```python
from build123d import *

# Parameters (mm, degrees)
F0_R     = 1.5
F1_DEPTH = 62
F2_W     = 60.3578643763
F2_H     = 56
F2_W_2   = 59.6421356237
F3_DEPTH = 100
F5_DEPTH = 3
F8_DEPTH = 3


with BuildPart() as f1:
    # F0 (on Front) → F1 (new body)
    with BuildSketch(Plane.XZ):
        with BuildLine():
            ThreePointArc((-3.5355339059, 3.5355339059), (0, 2.0710678119), (3.5355339059, 3.5355339059))
            Line((3.5355339059, 3.5355339059), (44, 44))
            Line((44, 44), (94.5, 44))
            ThreePointArc((94.5, 44), (98.0355339059, 45.4644660941), (99.5, 49))
            Line((99.5, 49), (99.5, 54))
            Line((99.5, 54), (39.8578643763, 54))
            Line((39.8578643763, 54), (-3.5355339059, 10.6066017178))
            ThreePointArc((-3.5355339059, 10.6066017178), (-5, 7.0710678119), (-3.5355339059, 3.5355339059))
        make_face()
        with Locations((0, 7.0710678119)):
            Circle(F0_R, mode=Mode.SUBTRACT)
        with Locations((12, 19.0710678119)):
            Circle(F0_R, mode=Mode.SUBTRACT)
    extrude(amount=F1_DEPTH)

    # F2 (on face) → F3 (cut)
    with BuildSketch(Plane.XY.offset(54)):
        with Locations((9.6789321881, -31)):
            Rectangle(F2_W, F2_H)
        with Locations((69.6789321881, -31)):
            Rectangle(F2_W_2, F2_H)
    extrude(amount=-F3_DEPTH, mode=Mode.SUBTRACT)


with BuildPart() as f5:
    # F4 (on face) → F5 (new body)
    with BuildSketch(Plane.XY.offset(54)):
        with BuildLine():
            ThreePointArc((99.5, -69), (92, -61.5), (84.5, -69))
            ThreePointArc((84.5, -69), (86.0313318068, -73.5414755311), (90, -76.2284161474))
            Line((90, -76.2284161474), (90, -74.123475383))
            ThreePointArc((90, -74.123475383), (88.8975815885, -64.4585244689), (97.5, -69))
            ThreePointArc((97.5, -69), (96.5414755311, -72.1024184115), (94, -74.123475383))
            Line((94, -74.123475383), (94, -76.2284161474))
            ThreePointArc((94, -76.2284161474), (97.9686681932, -73.5414755311), (99.5, -69))
        make_face()
        with BuildLine():
            ThreePointArc((89.3074175964, 0), (85.8175907598, 2.7540824329), (84.5, 7))
            Line((84.5, 7), (84.5, 0))
            Line((84.5, 0), (89.3074175964, 0))
        make_face()
        with BuildLine():
            Line((99.5, -3), (84.5, -3))
            Line((84.5, -3), (84.5, -69))
            ThreePointArc((84.5, -69), (92, -61.5), (99.5, -69))
            Line((99.5, -69), (99.5, -3))
        make_face()
        with BuildLine():
            ThreePointArc((99.5, 7), (98.1824092402, 2.7540824329), (94.6925824036, 0))
            Line((94.6925824036, 0), (99.5, 0))
            Line((99.5, 0), (99.5, 7))
        make_face()
        with BuildLine():
            Line((94.6925824036, 0), (89.3074175964, 0))
            ThreePointArc((89.3074175964, 0), (92, -0.5), (94.6925824036, 0))
        make_face()
        with BuildLine():
            ThreePointArc((90, 14.2284161474), (86.0313318068, 11.5414755311), (84.5, 7))
            ThreePointArc((84.5, 7), (85.8175907598, 2.7540824329), (89.3074175964, 0))
            Line((89.3074175964, 0), (94.6925824036, 0))
            ThreePointArc((94.6925824036, 0), (98.1824092402, 2.7540824329), (99.5, 7))
            ThreePointArc((99.5, 7), (97.9686681932, 11.5414755311), (94, 14.2284161474))
            Line((94, 14.2284161474), (94, 12.123475383))
            ThreePointArc((94, 12.123475383), (96.5414755311, 10.1024184115), (97.5, 7))
            ThreePointArc((97.5, 7), (88.8975815885, 2.4585244689), (90, 12.123475383))
            Line((90, 12.123475383), (90, 14.2284161474))
        make_face()
        with BuildLine():
            Line((89.3074175964, 0), (84.5, 0))
            Line((84.5, 0), (84.5, -3))
            Line((84.5, -3), (99.5, -3))
            Line((99.5, -3), (99.5, 0))
            Line((99.5, 0), (94.6925824036, 0))
            ThreePointArc((94.6925824036, 0), (92, -0.5), (89.3074175964, 0))
        make_face()
    extrude(amount=-F5_DEPTH)


with BuildPart() as f1_1:
    add(f1.part)

    # F6: union F5
    add(f5.part)

    # F7 (on face) → F8 (join)
    with BuildSketch(Plane.XY.offset(54)):
        with BuildLine():
            ThreePointArc((90, 12.123475383), (92, 1.5), (94, 12.123475383))
            Line((94, 12.123475383), (94, 9.8722813233))
            ThreePointArc((94, 9.8722813233), (95.1024184115, 8.6201851746), (95.5, 7))
            ThreePointArc((95.5, 7), (90.3798148254, 3.8975815885), (90, 9.8722813233))
            Line((90, 9.8722813233), (90, 12.123475383))
        make_face()
        with BuildLine():
            ThreePointArc((84.5, 7), (92, -0.5), (99.5, 7))
            ThreePointArc((99.5, 7), (97.9686681932, 11.5414755311), (94, 14.2284161474))
            Line((94, 14.2284161474), (94, 12.123475383))
            ThreePointArc((94, 12.123475383), (92, 1.5), (90, 12.123475383))
            Line((90, 12.123475383), (90, 14.2284161474))
            ThreePointArc((90, 14.2284161474), (86.0313318068, 11.5414755311), (84.5, 7))
        make_face()
        with BuildLine():
            Line((94, -71.8722813233), (94, -74.123475383))
            ThreePointArc((94, -74.123475383), (92, -63.5), (90, -74.123475383))
            Line((90, -74.123475383), (90, -71.8722813233))
            ThreePointArc((90, -71.8722813233), (90.3798148254, -65.8975815885), (95.5, -69))
            ThreePointArc((95.5, -69), (95.1024184115, -70.6201851746), (94, -71.8722813233))
        make_face()
        with BuildLine():
            ThreePointArc((94, -76.2284161474), (97.9686681932, -73.5414755311), (99.5, -69))
            ThreePointArc((99.5, -69), (92, -61.5), (84.5, -69))
            ThreePointArc((84.5, -69), (86.0313318068, -73.5414755311), (90, -76.2284161474))
            Line((90, -76.2284161474), (90, -74.123475383))
            ThreePointArc((90, -74.123475383), (92, -63.5), (94, -74.123475383))
            Line((94, -74.123475383), (94, -76.2284161474))
        make_face()
    extrude(amount=F8_DEPTH)


solid = f1_1.part
```
Verification items for the finished model (mm, model axes). A direction names the side the tool comes from. Round coordinates to 2 decimals unless told otherwise and drop trailing zeros. Order: outer loops, then holes, each group sorted by start corner. A loop starts at its lowest first (then second) coordinate and runs counter-clockwise, first axis right, second up. Notation, with made-up numbers: (60, 14.25) - (115, 14.25) arc R22 cw to (115, 53.25) - close; hole circle Ø1 at (19, 10). An arc over 180 degrees is marked (long way). Use CSV: the item, a comma, the result in double quotes.
(1) Mould release check, pull along Y, two halves, no side actions. Record for faces 1 (the face through (92, -65, 54)), 2 (the face through (69, -60, 44)): released by +Y, released by -Y, zero draft, split by the parting line, or undercut.
Entries:
face 1,"undercut"
face 2,"zero draft"
(2) Section check C-C on x = 12. Record the boundary of the cut face in (y, z).
Entries:
outline,"(-62, 12) - (-59, 12) - (-59, 17.57) - (-62, 17.57) - close; (-62, 20.57) - (-59, 20.57) - (-59, 26.14) - (-62, 26.14) - close; (-3, 12) - (0, 12) - (0, 17.57) - (-3, 17.57) - close; (-3, 20.57) - (0, 20.57) - (0, 26.14) - (-3, 26.14) - close"
(3) Section check A-A on x = 52. Record the boundary of the cut face in (y, z).
Entries:
outline,"(-62, 44) - (-59, 44) - (-59, 54) - (-62, 54) - close; (-3, 44) - (0, 44) - (0, 54) - (-3, 54) - close"
(4) Section check B-B on z = 46. Record the boundary of the cut face in (x, y).
Entries:
outline,"(31.86, -62) - (98.5, -62) - (98.5, -59) - (31.86, -59) - close; (31.86, -3) - (98.5, -3) - (98.5, 0) - (31.86, 0) - close"
(5) Section check D-D on x = 92. Record the boundary of the cut face in (y, z), and give its area (3 significant figures).
Entries:
outline,"(-65.5, 54) - (-63.5, 54) - (-63.5, 51) - (-62, 51) - (-62, 44) - (-59, 44) - (-59, 51) - (-3, 51) - (-3, 44) - (0, 44) - (0, 51) - (1.5, 51) - (1.5, 54) - (3.5, 54) - (3.5, 57) - (-0.5, 57) - (-0.5, 54) - (-61.5, 54) - (-61.5, 57) - (-65.5, 57) - close"
area,"261 mm^2"
(6) Access from +Z, -Z, +X, -X, +Y, -Y to the whole of each face (thin tool, end or side, straight path). Record for faces 3 (the face through (94, 13, 55)), 4 (the face through (69, -1, 44)), 5 (the face through (84.5, 4, 53)), 6 (the face through (95.91, -75.4, 54.71)).
Entries:
face 3,"+Z, -Z, +Y"
face 4,"-Z, +X, +Y, -Y"
face 5,"+Z, -Z, -X, +Y"
face 6,"+Z"
(7) Gauge pin test, flat ends, axial feed: pin 1 Ø3.5 at (y, z) = (12, 55) entering from +X; pin 2 Ø3.5 at (x, z) = (0, 7.07) entering from -Y; pin 3 Ø1.3 at (y, z) = (-75, 53.5) entering from -X; pin 4 Ø2.5 at (x, z) = (0, 7.07) entering from +Y. Record the tip position at first contact, or that the pin passes through.
Entries:
pin 1,"x = 98.76"
pin 2,"y = -62"
pin 3,"x = 86.74"
pin 4,"through"
(8) Thickness scan on probe 1 along Y at (x, z) = (68.5, 47.5); probe 2 along Y at (x, z) = (92, 55.7); probe 3 along X at (y, z) = (-4.5, 51.5). Record the ranges inside material, lowest first. Write a range as from..to.
Entries:
probe 1,"-62..-59, -3..0"
probe 2,"-65.5..-61.5, -0.5..3.5"
probe 3,"84.5..99.5"
